from build123d import *

# Parameters (mm, degrees)
BOSS_EXTRUDE1_DEPTH = 3
SKETCH2_R           = 4.5
SKETCH2_W           = 71.2
SKETCH2_H           = 24
SKETCH2_W_2         = 40
SKETCH2_H_2         = 10
CUT_EXTRUDE1_DEPTH  = 3


with BuildPart() as part:
    # Sketch1 → Boss-Extrude1 (new body)
    with BuildSketch(Plane(origin=(0, 0, 0), x_dir=(0, 0, -1), z_dir=(1, 0, 0))):
        Polygon((-46.800460417, 37.069263333), (-46.800460417, 19.294263333), (-43.800460417, 19.294263333), (-43.800460417, 5.044263333), (-46.800460417, 5.044263333), (-46.800460417, -9.205736667), (-43.800460417, -9.205736667), (-43.800460417, -23.455736667), (-46.800460417, -23.455736667), (-46.800460417, -37.705736667), (-46.800460417, -41.230736667), (-36.925460417, -41.230736667), (-36.925460417, -38.230736667), (-22.675460417, -38.230736667), (-22.675460417, -41.230736667), (-8.425460417, -41.230736667), (-8.425460417, -38.230736667), (5.824539583, -38.230736667), (5.824539583, -41.230736667), (20.074539583, -41.230736667), (20.074539583, -38.230736667), (34.324539583, -38.230736667), (34.324539583, -41.230736667), (44.199539583, -41.230736667), (44.199539583, -23.455736667), (41.199539583, -23.455736667), (41.199539583, -9.205736667), (44.199539583, -9.205736667), (44.199539583, 5.044263333), (41.199539583, 5.044263333), (41.199539583, 19.294263333), (44.199539583, 19.294263333), (44.199539583, 33.544263333), (44.199539583, 37.069263333), (34.324539583, 37.069263333), (34.324539583, 34.069263333), (20.074539583, 34.069263333), (20.074539583, 37.069263333), (5.824539583, 37.069263333), (5.824539583, 34.069263333), (-8.425460417, 34.069263333), (-8.425460417, 37.069263333), (-22.675460417, 37.069263333), (-22.675460417, 34.069263333), (-36.925460417, 34.069263333), (-36.925460417, 37.069263333), align=None)
    extrude(amount=BOSS_EXTRUDE1_DEPTH)

    # Sketch2 → Cut-Extrude1 (cut)
    with BuildSketch(Plane(origin=(3, 0, 0), x_dir=(0, 0, -1), z_dir=(1, 0, 0))):
        with Locations((20.094295928, -12.405736667)):
            Circle(SKETCH2_R)
        with Locations((7.989052272, -12.405736667)):
            Circle(SKETCH2_R)
        with Locations(Location((31.989052272, -12.405736667, 0), (0, 0, 180))):
            Circle(SKETCH2_R)
        with Locations((-3.200460417, 16.569263333)):
            Rectangle(SKETCH2_W, SKETCH2_H)
        with Locations((-21.800460417, -28.230736667)):
            Rectangle(SKETCH2_W_2, SKETCH2_H_2)
    extrude(amount=-CUT_EXTRUDE1_DEPTH, mode=Mode.SUBTRACT)


solid = part.part
Geometry: final body of the model. Coordinates: model frame, mm. A direction names the side the tool comes from. Round coordinates to 2 decimals unless told otherwise and drop trailing zeros. Loops run counter-clockwise (first coordinate to the right, second up) from the corner with the lowest first, then second, coordinate; pieces in that order, holes last.
Q1. Pin query (flat end, axial travel): P1, Ø0.9, axis at x = 1.5, y = -17, coming from the -Z side; P2, Ø1, axis at x = 1, z = -33, coming from the -Y side. Return the tip coordinate at first contact, or that it passes through.
Q2. Access query for faces 1 (the flat face through (1, 5.044, 45)), 2 (the flat face through (1, -38.231, 1)), 3 (the flat face through (1, 36, -20.075)). Directions: +Z, -Z, +X, -X, +Y, -Y. A direction counts if a zero-diameter tool reaches every point of the face in a straight line with its end or side. Return the directions, or none.
Q3. Section C-C on y = 10.5. Return loops of the section in (x, z), plus the area to 3 significant figures.
Q4. Section D-D on z = 11.5. Return loops of the section in (x, y), plus the area to 3 significant figures.
Q5. Section B-B on z = 31. Return loops of the section in (x, y).
Q6. Pull-direction query (Y, two-part tool) for faces 4 (the flat face through (1, -38.231, 30)), 5 (the flat face through (2, -28, 41.8)), 6 (the flat face through (1, 36, -34.325)); classes: released by +Y, released by -Y, zero draft, split by the parting line, or undercut.
Q7. Material intervals for L1, parallel to Y at x = 1, z = 6.5; L2, parallel to Y at x = 2.05, z = 15.5; L3, parallel to Y at x = 2.4, z = 39, sorted ascending.
Q8. Section A-A on y = -25.5. Return loops of the section in (x, z), plus the area to 3 significant figures.
Evaluation:
1. P1: stops at z = -41.2
1. P2: stops at y = -38.23
2. face 1: +Z, +X, -X
2. face 2: +X, -X, -Y
2. face 3: +X, -X, +Y
3. outline: (0, -41.2) - (3, -41.2) - (3, -32.4) - (0, -32.4) - close; (0, 38.8) - (3, 38.8) - (3, 43.8) - (0, 43.8) - close
3. area: 41.4 mm2
4. outline: (0, -41.23) - (3, -41.23) - (3, -33.23) - (0, -33.23) - close; (0, -23.23) - (3, -23.23) - (3, 4.57) - (0, 4.57) - close; (0, 28.57) - (3, 28.57) - (3, 37.07) - (0, 37.07) - close
4. area: 133 mm2
5. outline: (0, -38.23) - (3, -38.23) - (3, -33.23) - (0, -33.23) - close; (0, -23.23) - (3, -23.23) - (3, 4.57) - (0, 4.57) - close; (0, 28.57) - (3, 28.57) - (3, 34.07) - (0, 34.07) - close
6. face 4: released by -Y
6. face 5: undercut
6. face 6: zero draft
7. L1: y = -38.23 to -33.23, -23.23 to 4.57, 28.57 to 34.07
7. L2: y = -41.23 to -33.23, -23.23 to 4.57, 28.57 to 37.07
7. L3: y = -41.23 to -33.23, -23.23 to 37.07
8. outline: (0, -44.2) - (3, -44.2) - (3, 1.8) - (0, 1.8) - close; (0, 41.8) - (3, 41.8) - (3, 46.8) - (0, 46.8) - close
8. area: 153 mm2
